Source: CAD feature listing. Evaluate the final solid. Frame: model axes, mm. Face numbers are marked on the shaded views. A direction names the side the tool comes from. Give positions to 0.01 mm unless a question says otherwise; leave off trailing zeros. Order: outer loops, then holes, each group sorted by start corner. A loop starts at its lowest first (then second) coordinate and runs counter-clockwise, first axis right, second up.
1) Section B-B, the plane y = 0. Return loops of the section in (x, z), plus the area to 3 significant figures.
2) Draft query along Y for the marked faces 4, 5, 6 and 7. Return one class per face: released by +Y, released by -Y, zero draft, split by the parting line, or undercut.
3) First-contact query: P1, Ø2, axis at x = 12, y = -31, coming from the -Z side; P2, Ø1, axis at y = -18.5, z = 4, coming from the -X side; P3, Ø4, axis at x = 28.5, z = 13, coming from the +Y side. Flat tips, straight axial feed; report the tip coordinate or a pass-through.
4) Section A-A, the plane x = 0. Return loops of the section in (y, z), plus the area to 3 significant figures.
5) Material intervals for line 1 (Y direction, x = 21, z = 17); line 2 (Z direction, x = -16, y = 3.5); line 3 (X direction, y = -9, z = 15), sorted ascending.
6) Access query for the marked faces 1, 2 and 3. Directions: +Z, -Z, +X, -X, +Y, -Y. A direction counts if a zero-diameter tool reaches every point of the face in a straight line with its end or side. Return the directions, or none.
```python
from build123d import *

# Parameters (mm, degrees)
F3_W           = 8.3933982822
F3_H           = 16.3933982822
F4_ANGLE_BACK  = 70
F4_ANGLE       = 140
F6_ANGLE_START = 100
F6_ANGLE       = 160
F7_ANGLE_BACK  = 70
F7_ANGLE       = 140
F8_R           = 3
F8_2_R         = 3
F9_R           = 3
F13_DEPTH      = 10
F14_R          = 22
F15_DEPTH      = 1.5


with BuildPart() as f1:
    # F0 (on Front) → F1 (revolve)
    with BuildSketch(Plane.XZ):
        Polygon((-43.5, 14.5), (-27, -2), (0, -2), (0, 20), (-44, 20), (-44, 16), (-43.5, 15.5), align=None)
    revolve(axis=Axis((0, 0, 9.4880101401), (0, 0, -1)))


with BuildPart() as f4:
    # F3 (on Front) → F4 (revolve)
    with BuildSketch(Plane.XZ, mode=Mode.PRIVATE) as f4_sk:
        with Locations((-41.8033008589, 16.8033008589)):
            Rectangle(F3_W, F3_H)
    revolve(f4_sk.sketch.rotate(Axis((0, 0, 9.4880101401), (0, 0, -1)), -F4_ANGLE_BACK), axis=Axis((0, 0, 9.4880101401), (0, 0, -1)), revolution_arc=F4_ANGLE)

    # F8#2
    f8_2_edges = [f4.edges().sort_by_distance(p)[0] for p in [
        (-12.862215, 35.338646, 16.803301),
        (-12.862215, -35.338646, 16.803301),
    ]]
    fillet(f8_2_edges, radius=F8_2_R)


with BuildPart() as f6:
    # F5 (on Front) → F6 (revolve)
    with BuildSketch(Plane.XZ, mode=Mode.PRIVATE) as f6_sk:
        Polygon((-36.8994949366, -6.2426406871), (-25.5857864376, 5.0710678119), (-37.6066017178, 17.091883092), (-48.9203102168, 5.7781745931), align=None)
    revolve(f6_sk.sketch.rotate(Axis((0, 0, 9), (0, 0, -1)), F6_ANGLE_START), axis=Axis((0, 0, 9), (0, 0, -1)), revolution_arc=F6_ANGLE)

    # F9
    f9_edges = [f6.edges().sort_by_distance(p)[0] for p in [
        (5.425228, 30.767995, -0.585786),
        (7.51262, 42.606187, 11.435029),
        (7.51262, -42.606187, 11.435029),
        (5.425228, -30.767995, -0.585786),
    ]]
    fillet(f9_edges, radius=F9_R)


with BuildPart() as f7:
    # F2 (on Front) → F7 (revolve)
    with BuildSketch(Plane.XZ, mode=Mode.PRIVATE) as f7_sk:
        Polygon((-41.2877159425, 2.0970603683), (-31.9497474683, 11.4350288425), (-37.6066017178, 17.091883092), (-46.944570192, 7.7539146178), align=None)
    revolve(f7_sk.sketch.rotate(Axis((0, 0, 9), (0, 0, -1)), -F7_ANGLE_BACK), axis=Axis((0, 0, 9), (0, 0, -1)), revolution_arc=F7_ANGLE)

    # F8
    f8_edges = [f7.edges().sort_by_distance(p)[0] for p in [
        (-12.524344, -34.410352, 6.766045),
        (-12.524344, 34.410352, 6.766045),
    ]]
    fillet(f8_edges, radius=F8_R)


with BuildPart() as f1_1:
    add(f1.part)

    # F10: cut F7, F4, F6
    add(f7.part, mode=Mode.SUBTRACT)
    add(f4.part, mode=Mode.SUBTRACT)
    add(f6.part, mode=Mode.SUBTRACT)

    # F12 (on offset) → F13 (cut)
    with BuildSketch(Plane(origin=(0, 0, -2), x_dir=(1, 0, 0), z_dir=(0, 0, -1))):
        with BuildLine():
            ThreePointArc((-11, 2.5), (-13.5, 0), (-11, -2.5))
            Line((-11, -2.5), (0, -2.5))
            Line((0, -2.5), (11, -2.5))
            ThreePointArc((11, -2.5), (13.5, 0), (11, 2.5))
            Line((11, 2.5), (0, 2.5))
            Line((0, 2.5), (-11, 2.5))
        make_face()
    extrude(amount=-F13_DEPTH, mode=Mode.SUBTRACT)

    # F14 (on offset) → F15 (cut)
    with BuildSketch(Plane(origin=(0, 0, -2), x_dir=(1, 0, 0), z_dir=(0, 0, -1))):
        Circle(F14_R)
    extrude(amount=-F15_DEPTH, mode=Mode.SUBTRACT)


solid = f1_1.part
```
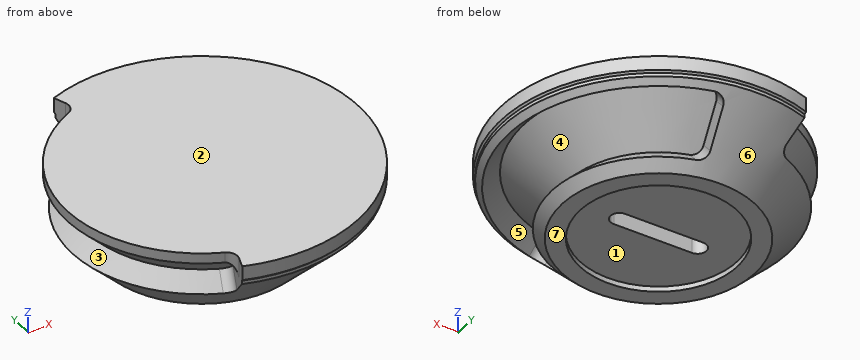
From the geometry:
1. outline: (-37.61, 17.09) - (-31.95, 11.44) - (-36.19, 7.19) - (-27, -2) - (-22, -2) - (-22, -0.5) - (-13.5, -0.5) - (-13.5, 8) - (13.5, 8) - (13.5, -0.5) - (22, -0.5) - (22, -2) - (27, -2) - (29.83, 0.83) - (25.59, 5.07) - (37.61, 17.09) - (41.85, 12.85) - (43.5, 14.5) - (43.5, 15.5) - (44, 16) - (44, 20) - (-37.61, 20) - close
1. area: 1,170 mm2
2. face 4: undercut
2. face 5: undercut
2. face 6: split by the parting line
2. face 7: zero draft
3. P1: stops at z = 11.73
3. P2: stops at x = -28.01
3. P3: stops at y = 33.97
4. outline: (-44, 16) - (-43.5, 15.5) - (-43.5, 14.5) - (-27, -2) - (-22, -2) - (-22, -0.5) - (-2.5, -0.5) - (-2.5, 8) - (2.5, 8) - (2.5, -0.5) - (22, -0.5) - (22, -2) - (27, -2) - (43.5, 14.5) - (43.5, 15.5) - (44, 16) - (44, 20) - (-44, 20) - close
4. area: 1,540 mm2
5. line 1: y = -38.67 to -31.31, -31.09 to 31.09, 31.31 to 38.67
5. line 2: z = -0.5 to 20
5. line 3: x = -34.36 to 34.36, 38.66 to 42.56
6. face 1: -Z
6. face 2: +Z, +X, -X, +Y, -Y
6. face 3: -X
